Work out the finished part from the listing and answer in its coordinate system (mm). A direction names the side the tool comes from. Round coordinates to 2 decimals unless told otherwise and drop trailing zeros. Write each loop counter-clockwise with the first axis right and the second up, starting at its lowest first coordinate (ties: lowest second). Pieces come first, ordered by that corner, then holes.
1. Straight lines are drawn through the part: probe 1 along X at (y, z) = (2.4, -8.5); probe 2 along Z at (x, y) = (-18, 2.2); probe 3 along X at (y, z) = (2.1, 28.5). For each, find the intervals that lie inside material, in ascending order.
2. Find section C-C (z = -54). Write down the section's boundary in (x, y).
3. A tool of negligible diameter and unlimited length cuts with its end or side. For faces 4 (the face through (-12.55, 1.48, -85.72)), 5 (the face through (-108, 1.52, 108.07)), 6 (the face through (81.462, 1.479, 98.095)), from which of +Z, -Z, +X, -X, +Y, -Y can it reach the whole face along a straight path? Write none if from no direction.
4. Determine the mould class of faces 1 (the face through (-2, 0, -26)), 2 (the face through (70.305, 1.479, -82.534)), 3 (the face through (-108.07, 1.52, -108)) for opening direction X: pulls with the +X half, pulls with the -X half, needs draft (parallel to the pull), parting line crosses it, or undercut.
5. Find section A-A (z = 54.5). Write down the section's boundary in (x, y).
6. Find section B-B (x = -28). Write down the section's boundary in (y, z).
7. Find section D-D (y = 2.45). Count the separate pieces of the cut face and the enclosed holes in it, and give its area (3 significant figures).
```python
from build123d import *

# Parameters (mm, degrees)
SKETCH1_R           = 1.7
SKETCH1_R_2         = 2.25
SKETCH1_R_3         = 1.65
BOSS_EXTRUDE1_DEPTH = 3
FILLET1_R           = 5


with BuildPart() as part:
    # Sketch1 → Boss-Extrude1 (new body)
    with BuildSketch(Plane(origin=(0, 0, 0), x_dir=(1, 0, 0), z_dir=(0, 1, 0))):
        Polygon((-99.587138739, -109.5), (-61.5, -85.533985256), (-61.5, -15), (61.5, -15), (61.5, -85.533985256), (99.587138739, -109.5), (109.5, -109.5), (109.5, 109.5), (-109.5, 109.5), (-109.5, -109.5), align=None)
        with Locations(Location((-104.5, 104.5, 0), (0, 0, 270))):
            Circle(SKETCH1_R, mode=Mode.SUBTRACT)
        with Locations(Location((104.5, 104.5, 0), (0, 0, 270))):
            Circle(SKETCH1_R, mode=Mode.SUBTRACT)
        with Locations(Location((104.5, -104.5, 0), (0, 0, 90))):
            Circle(SKETCH1_R, mode=Mode.SUBTRACT)
        with Locations(Location((-104.5, -104.5, 0), (0, 0, 90))):
            Circle(SKETCH1_R, mode=Mode.SUBTRACT)
        with Locations(Location((-97, 9, 0), (0, 0, 270))):
            Circle(SKETCH1_R_2, mode=Mode.SUBTRACT)
        with Locations(Location((-73, 9, 0), (0, 0, 270))):
            Circle(SKETCH1_R_2, mode=Mode.SUBTRACT)
        with Locations(Location((-73, -9, 0), (0, 0, 270))):
            Circle(SKETCH1_R_2, mode=Mode.SUBTRACT)
        with Locations(Location((-97, -9, 0), (0, 0, 270))):
            Circle(SKETCH1_R_2, mode=Mode.SUBTRACT)
        with Locations(Location((-97, 46.5, 0), (0, 0, 270))):
            Circle(SKETCH1_R_2, mode=Mode.SUBTRACT)
        with Locations(Location((-73, 46.5, 0), (0, 0, 270))):
            Circle(SKETCH1_R_2, mode=Mode.SUBTRACT)
        with Locations(Location((-73, 28.5, 0), (0, 0, 270))):
            Circle(SKETCH1_R_2, mode=Mode.SUBTRACT)
        with Locations(Location((-97, 28.5, 0), (0, 0, 270))):
            Circle(SKETCH1_R_2, mode=Mode.SUBTRACT)
        with Locations(Location((-97, -28.5, 0), (0, 0, 90))):
            Circle(SKETCH1_R_2, mode=Mode.SUBTRACT)
        with Locations(Location((-73, -28.5, 0), (0, 0, 90))):
            Circle(SKETCH1_R_2, mode=Mode.SUBTRACT)
        with Locations(Location((-73, -46.5, 0), (0, 0, 90))):
            Circle(SKETCH1_R_2, mode=Mode.SUBTRACT)
        with Locations(Location((-97, -46.5, 0), (0, 0, 90))):
            Circle(SKETCH1_R_2, mode=Mode.SUBTRACT)
        with Locations(Location((73, -46.5, 0), (0, 0, 270))):
            Circle(SKETCH1_R_2, mode=Mode.SUBTRACT)
        with Locations(Location((97, -46.5, 0), (0, 0, 270))):
            Circle(SKETCH1_R_2, mode=Mode.SUBTRACT)
        with Locations(Location((73, -28.5, 0), (0, 0, 270))):
            Circle(SKETCH1_R_2, mode=Mode.SUBTRACT)
        with Locations(Location((97, -28.5, 0), (0, 0, 270))):
            Circle(SKETCH1_R_2, mode=Mode.SUBTRACT)
        with Locations(Location((73, 28.5, 0), (0, 0, 90))):
            Circle(SKETCH1_R_2, mode=Mode.SUBTRACT)
        with Locations(Location((97, 28.5, 0), (0, 0, 90))):
            Circle(SKETCH1_R_2, mode=Mode.SUBTRACT)
        with Locations(Location((73, 46.5, 0), (0, 0, 90))):
            Circle(SKETCH1_R_2, mode=Mode.SUBTRACT)
        with Locations(Location((97, 46.5, 0), (0, 0, 90))):
            Circle(SKETCH1_R_2, mode=Mode.SUBTRACT)
        with Locations(Location((0, 104.5, 0), (0, 0, 270))):
            Circle(SKETCH1_R, mode=Mode.SUBTRACT)
        with Locations(Location((104.5, 0, 0), (0, 0, 270))):
            Circle(SKETCH1_R, mode=Mode.SUBTRACT)
        with Locations(Location((-6, 8.81582657, 0), (0, 0, 270))):
            Circle(SKETCH1_R_3, mode=Mode.SUBTRACT)
        with Locations(Location((6, 8.81582657, 0), (0, 0, 270))):
            Circle(SKETCH1_R_3, mode=Mode.SUBTRACT)
        with Locations(Location((6, -11.18417343, 0), (0, 0, 270))):
            Circle(SKETCH1_R_3, mode=Mode.SUBTRACT)
        with Locations(Location((-6, -11.18417343, 0), (0, 0, 270))):
            Circle(SKETCH1_R_3, mode=Mode.SUBTRACT)
        with BuildLine():
            Line((-10.147064808, 80.005570394), (-10.147064808, 44.141462897))
            ThreePointArc((-10.147064808, 44.141462897), (-14.691860424, 36.926093006), (-23.162455474, 37.908818476))
            Line((-23.162455474, 37.908818476), (-67.730913723, 73.772925974))
            ThreePointArc((-67.730913723, 73.772925974), (-70.260758486, 82.664408922), (-62.715523057, 88.005570394))
            Line((-62.715523057, 88.005570394), (-18.147064808, 88.005570394))
            ThreePointArc((-18.147064808, 88.005570394), (-12.490210559, 85.662424644), (-10.147064808, 80.005570394))
        make_face(mode=Mode.SUBTRACT)
        with BuildLine():
            Line((10.147064808, 80.005570394), (10.147064808, 44.141462897))
            ThreePointArc((10.147064808, 44.141462897), (14.691860424, 36.926093006), (23.162455474, 37.908818476))
            Line((23.162455474, 37.908818476), (67.730913723, 73.772925974))
            ThreePointArc((67.730913723, 73.772925974), (70.260758486, 82.664408922), (62.715523057, 88.005570394))
            Line((62.715523057, 88.005570394), (18.147064808, 88.005570394))
            ThreePointArc((18.147064808, 88.005570394), (12.490210559, 85.662424644), (10.147064808, 80.005570394))
        make_face(mode=Mode.SUBTRACT)
    extrude(amount=BOSS_EXTRUDE1_DEPTH)

    # Fillet1
    fillet1_edges = [part.edges().sort_by_distance(p)[0] for p in [
        (109.5, 1.5, 109.5),
        (61.5, 1.5, 85.533985256),
        (61.5, 1.5, 15),
        (-61.5, 1.5, 15),
        (-61.5, 1.5, 85.533985256),
        (-99.587138739, 1.5, 109.5),
        (-109.5, 1.5, 109.5),
        (-109.5, 1.5, -109.5),
        (109.5, 1.5, -109.5),
    ]]
    fillet(fillet1_edges, radius=FILLET1_R)


solid = part.part
```
Worked answers:
1. probe 1: x = -109.5 to -99.19, -94.81 to -75.19, -70.81 to -7.62, -4.38 to 4.38, 7.62 to 109.5
1. probe 2: z = -109.5 to -88, -36.14 to 15
1. probe 3: x = -109.5 to -99.25, -94.75 to -75.25, -70.75 to -61.5, 61.5 to 70.75, 75.25 to 94.75, 99.25 to 109.5
2. outline: (-109.5, 0) - (-43.16, 0) - (-43.16, 3) - (-109.5, 3) - close; (-10.15, 0) - (10.15, 0) - (10.15, 3) - (-10.15, 3) - close; (43.16, 0) - (109.5, 0) - (109.5, 3) - (43.16, 3) - close
3. face 4: +Y, -Y
3. face 5: +Z, -X, +Y, -Y
3. face 6: +Z, +Y, -Y
4. face 1: needs draft
4. face 2: undercut
4. face 3: pulls with the -X half
5. outline: (-109.5, 0) - (-61.5, 0) - (-61.5, 3) - (-109.5, 3) - close; (61.5, 0) - (109.5, 0) - (109.5, 3) - (61.5, 3) - close
6. outline: (0, -109.5) - (3, -109.5) - (3, -88.01) - (0, -88.01) - close; (0, -41.8) - (3, -41.8) - (3, 15) - (0, 15) - close
7. separate pieces: 1
7. enclosed holes: 32
7. area: 30,800 mm2
